from build123d import *

# Parameters (mm, degrees)
F0_R           = 15
F1_DEPTH       = 8
F3_D           = 4.4
F3_CSINK_D     = 8.96
F3_CSINK_ANGLE = 90
F5_D           = 5.5
F5_CSINK_D     = 11.2
F5_CSINK_ANGLE = 90
F6_R           = 5


with BuildPart() as f1:
    # F0 (on Front) → F1 (new body)
    with BuildSketch(Plane.XZ):
        with BuildLine():
            Line((-44.9550832745, 65.1504273235), (-58.4898427156, 65.1504273235))
            ThreePointArc((-58.4898427156, 65.1504273235), (-62.9799707761, 63.290555384), (-64.8398427156, 58.8004273235))
            Line((-64.8398427156, 58.8004273235), (-64.8398427156, 44.9648132355))
            ThreePointArc((-64.8398427156, 44.9648132355), (-64.5186166173, 43.2015563694), (-63.5962128052, 41.6648611525))
            Line((-63.5962128052, 41.6648611525), (-61.8242943859, 39.6478678193))
            ThreePointArc((-61.8242943859, 39.6478678193), (-46.8824791526, 0), (-61.8242943859, -39.6478678193))
            Line((-61.8242943859, -39.6478678193), (-63.5962128052, -41.6648611525))
            ThreePointArc((-63.5962128052, -41.6648611525), (-64.5186166173, -43.2015563694), (-64.8398427156, -44.9648132355))
            Line((-64.8398427156, -44.9648132355), (-64.8398427156, -58.4995726765))
            ThreePointArc((-64.8398427156, -58.4995726765), (-62.9799707761, -62.989700737), (-58.4898427156, -64.8495726765))
            Line((-58.4898427156, -64.8495726765), (-44.6542286275, -64.8495726765))
            ThreePointArc((-44.6542286275, -64.8495726765), (-42.8909717614, -64.5283465783), (-41.3542765446, -63.6059427661))
            Line((-41.3542765446, -63.6059427661), (-39.3372832113, -61.8340243469))
            ThreePointArc((-39.3372832113, -61.8340243469), (0.3105846079, -46.8922091135), (39.9584524272, -61.8340243469))
            Line((39.9584524272, -61.8340243469), (41.9754457605, -63.6059427661))
            ThreePointArc((41.9754457605, -63.6059427661), (43.5121409773, -64.5283465783), (45.2753978434, -64.8495726765))
            Line((45.2753978434, -64.8495726765), (58.8101572844, -64.8495726765))
            ThreePointArc((58.8101572844, -64.8495726765), (63.300285345, -62.989700737), (65.1601572844, -58.4995726765))
            Line((65.1601572844, -58.4995726765), (65.1601572844, -44.6639585885))
            ThreePointArc((65.1601572844, -44.6639585885), (64.8389311862, -42.9007017224), (63.9165273741, -41.3640065055))
            Line((63.9165273741, -41.3640065055), (62.1446089548, -39.3470131723))
            ThreePointArc((62.1446089548, -39.3470131723), (47.2027937215, 0.300854647), (62.1446089548, 39.9487224663))
            Line((62.1446089548, 39.9487224663), (63.9165273741, 41.9657157995))
            ThreePointArc((63.9165273741, 41.9657157995), (64.8389311862, 43.5024110164), (65.1601572844, 45.2656678825))
            Line((65.1601572844, 45.2656678825), (65.1601572844, 58.8004273235))
            ThreePointArc((65.1601572844, 58.8004273235), (63.300285345, 63.290555384), (58.8101572844, 65.1504273235))
            Line((58.8101572844, 65.1504273235), (44.9745431964, 65.1504273235))
            ThreePointArc((44.9745431964, 65.1504273235), (43.2112863303, 64.8292012253), (41.6745911135, 63.9067974131))
            Line((41.6745911135, 63.9067974131), (39.6575977802, 62.1348789939))
            ThreePointArc((39.6575977802, 62.1348789939), (0.0097299609, 47.1930637605), (-39.6381378583, 62.1348789939))
            Line((-39.6381378583, 62.1348789939), (-41.6551311916, 63.9067974131))
            ThreePointArc((-41.6551311916, 63.9067974131), (-43.1918264084, 64.8292012253), (-44.9550832745, 65.1504273235))
        make_face()
        with Locations((0.1601572844, 0.1504273235)):
            Circle(F0_R, mode=Mode.SUBTRACT)
    extrude(amount=F1_DEPTH)

    # F3 (through all)
    with Locations(Plane.XZ.offset(8)):
        with Locations((-50, 50.2785483839), (50, 50), (49.3192886108, -50), (-50, -50), (-37.5, 37.5), (37.5, 37.5), (37.5, -37.5), (-37.5, -37.5)):
            CounterSinkHole(F3_D / 2, F3_CSINK_D / 2, counter_sink_angle=F3_CSINK_ANGLE)

    # F5 (through all)
    with Locations(Plane(origin=(0, 0, 0), x_dir=(-1, 0, 0), z_dir=(0, 1, 0))):
        with Locations((0, -30), (0, 30)):
            CounterSinkHole(F5_D / 2, F5_CSINK_D / 2, counter_sink_angle=F5_CSINK_ANGLE)

    # F6
    f6_edges = [f1.edges().sort_by_distance(p)[0] for p in [
        (-51.572036, 0, -64.849573),
        (63.300285, 0, -62.989701),
        (65.160157, 0, 52.033048),
        (-62.979971, 0, -62.989701),
        (-64.839843, 0, 51.88262),
        (-62.979971, 0, 63.290555),
        (-51.722463, 0, 65.150427),
        (63.300285, 0, 63.290555),
        (-14.839843, 0, 0.150427),
    ]]
    fillet(f6_edges, radius=F6_R)


solid = f1.part
Work out the finished part from the listing and answer in its coordinate system (mm). A direction names the side the tool comes from. Give positions to 0.01 mm unless a question says otherwise; leave off trailing zeros. Answer as CSV lines item,"result".
Q1. A tool of negligible diameter and unlimited length cuts with its end or side. For faces 1 (the cylindrical face through (43.49, -6.48, -64.52)), 2 (the cylindrical face through (49.796, -2.82, -52.148)), 3 (the cylindrical face through (61.947, -1.504, -41.282)), from which of +Z, -Z, +X, -X, +Y, -Y can it reach the whole face along a straight path? Write none if from no direction.
A:
face 1,"-Z, +Y, -Y"
face 2,"+Y, -Y"
face 3,"+X, +Y"
Q2. The mould has two halves that part along X. Classify faces 4 (the cylindrical face through (63.25, -6.48, -63.04)), 5 (the cylindrical face through (41.593, -1.504, 61.937)), 6 (the cylindrical face through (-64.53, -6.48, 43.23)): +X half, -X half, draft (parallel to the pull), parting line (faces both ways), or undercut.
A:
face 4,"+X half"
face 5,"undercut"
face 6,"-X half"
Q3. Find the intervals of material crossed by probe 1 along Z at (x, y) = (0, -4.8); probe 2 along Z at (x, y) = (35.5, -3.5); probe 3 along X at (y, z) = (-3.75, 37.5), in increasing order. Write a range as [from, to].
A:
probe 1,"z = [-46.89, -32.75], [-27.25, -14.85], [15.15, 27.25], [32.75, 47.19]"
probe 2,"z = [-57.99, -38.42], [-36.58, 36.58], [38.42, 58.51]"
probe 3,"x = [-59.82, -39.7], [-35.3, 35.3], [39.7, 59.9]"
Q4. Given P1, Ø1.5, axis at x = -0.5, z = -44, coming from the +Y side; P2, Ø5, axis at x = 37.5, z = -37.5, coming from the -Y side; P3, Ø1.5, axis at x = 19.5, y = -1, coming from the -Z side, each flat-ended and moving along its own axis, determine where each tip first touches the part or whether it passes through.
A:
P1,"stops at y = -0.19"
P2,"stops at y = -6.02"
P3,"stops at z = -48.82"
Q5. A cutting plane is placed at A-A on z = -37.5. Count the separate pieces of the cut face and the enclosed holes in it, plus the area to 3 significant figures.
A:
separate pieces,"3"
enclosed holes,"0"
area,"870 mm²"
